```python
from build123d import *

# Parameters (mm, degrees)
F0_W      = 1066.8
F0_H      = 457.2
F1_DEPTH  = 50.8
F2_R      = 50.8
F3_SIZE   = 44.45
F4_W      = 939.8
F4_H      = 330.2
F5_DEPTH  = 25.4
F10_DEPTH = 19.05


with BuildPart() as f1:
    # F0 (on Top) → F1 (new body)
    with BuildSketch(Plane.XY):
        Rectangle(F0_W, F0_H)
    extrude(amount=-F1_DEPTH)

    # F2
    f2_edges = [f1.edges().sort_by_distance(p)[0] for p in [
        (-533.4, -228.6, -25.4),
        (-533.4, 228.6, -25.4),
        (533.4, -228.6, -25.4),
        (533.4, 228.6, -25.4),
    ]]
    fillet(f2_edges, radius=F2_R)

    # F3
    f3_edges = [f1.edges().sort_by_distance(p)[0] for p in [
        (533.4, 0, -50.8),
    ]]
    chamfer(f3_edges, length=F3_SIZE)

    # F4 (on face) → F5 (cut)
    with BuildSketch(Plane(origin=(0, 0, -50.8), x_dir=(1, 0, 0), z_dir=(0, 0, -1))):
        Rectangle(F4_W, F4_H)
    extrude(amount=-F5_DEPTH, mode=Mode.SUBTRACT)

    # F9 (on face) → F10 (join, symmetric)
    with BuildSketch(Plane(origin=(-38.1, 65.991136, 0), x_dir=(0.866025, 0.5, 0), z_dir=(0.5, -0.866025, 0))):
        Polygon((-409.78602, -736.6), (-284.382272, -25.4), (-385.982272, -25.4), (-460.58602, -736.6), align=None)
    extrude(amount=F10_DEPTH, both=True)

    # F11: F1 across plane


with BuildPart() as f1_1:
    add(f1.part)
    add(f1.part.mirror(Plane.YZ))

    # F12: F1 across plane


with BuildPart() as f1_2:
    add(f1_1.part)
    add(f1_1.part.mirror(Plane.XZ))


solid = f1_2.part
```
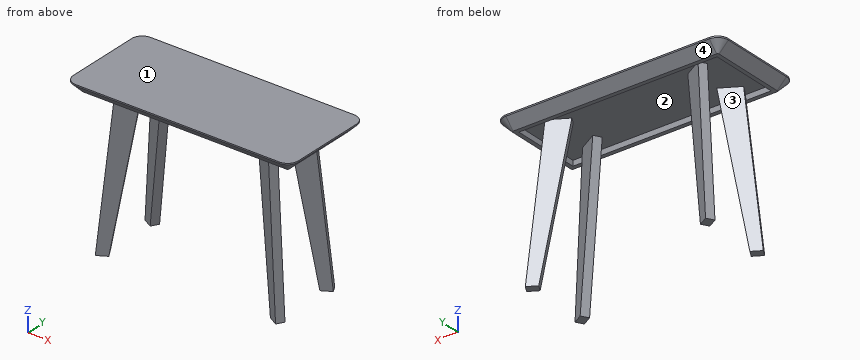
Geometry check sheet. Reference: the model listing, model coordinates, mm. Face numbers are marked on the shaded views. Give positions to 0.01 mm unless a question says otherwise; leave off trailing zeros. Write each loop counter-clockwise with the first axis right and the second up, starting at its lowest first coordinate (ties: lowest second). Pieces come first, ordered by that corner, then holes.
1) Section check D-D, the plane z = -508.5. Record the boundary of the cut face in (x, y).
2) Gauge pin test, flat ends, axial feed: pin 1 (10 mm diameter, centred on y = 115, z = -318, fed in from +X); pin 2 (20.5 mm diameter, centred on x = 157.5, z = -41, fed in from -Y); pin 3 (10 mm diameter, centred on y = -112, z = -191.5, fed in from +X). Record the tip position at first contact, or that the pin passes through.
3) Material ranges on L1, parallel to X at y = -80.5, z = -36; L2, parallel to Z at x = -213.5, y = -13.5; L3, parallel to X at y = 154.5, z = -322, recorded low to high.
4) Section check A-A, the plane x = 193.5. Record the boundary of the cut face in (y, z), and give its area (3 significant figures).
5) Section check B-B, the plane z = -263. Record the boundary of the cut face in (x, y), and give its area (3 significant figures).
6) Section check C-C, the plane y = 33.5. Record the boundary of the cut face in (x, z), and give its area (3 significant figures).
7) Release check for a two-part mould opening along Y. For the marked faces 1, 2, 3 and 4 record: pulls with the +Y half, pulls with the -Y half, needs draft (parallel to the pull), parting line crosses it, or undercut.
Computed:
1. outline: (-425.78, -135.84) - (-406.73, -168.84) - (-348.63, -135.29) - (-367.68, -102.29) - close; (-425.78, 135.84) - (-367.68, 102.29) - (-348.63, 135.29) - (-406.73, 168.84) - close; (348.63, -135.29) - (406.73, -168.84) - (425.78, -135.84) - (367.68, -102.29) - close; (348.63, 135.29) - (367.68, 102.29) - (425.78, 135.84) - (406.73, 168.84) - close
2. pin 1: stops at x = 398.35
2. pin 2: stops at y = -204.2
2. pin 3: stops at x = 393.15
3. L1: x = -503.75 to -469.9, -329.93 to -284.06, 284.06 to 329.93, 469.9 to 503.75
3. L2: z = -25.4 to 0
3. L3: x = -392.42 to -381.9, 381.9 to 392.42
4. outline: (-228.6, -6.35) - (-184.15, -50.8) - (-165.1, -50.8) - (-165.1, -25.4) - (165.1, -25.4) - (165.1, -50.8) - (184.15, -50.8) - (228.6, -6.35) - (228.6, 0) - (-228.6, 0) - close
4. area: 12,900 mm2
5. outline: (-403.48, -122.96) - (-384.43, -155.96) - (-311.14, -113.65) - (-330.19, -80.65) - close; (-403.48, 122.96) - (-330.19, 80.65) - (-311.14, 113.65) - (-384.43, 155.96) - close; (311.14, -113.65) - (384.43, -155.96) - (403.48, -122.96) - (330.19, -80.65) - close; (311.14, 113.65) - (330.19, 80.65) - (403.48, 122.96) - (384.43, 155.96) - close
5. area: 12,900 mm2
6. outline: (-533.4, -6.35) - (-488.95, -50.8) - (-469.9, -50.8) - (-469.9, -25.4) - (469.9, -25.4) - (469.9, -50.8) - (488.95, -50.8) - (533.4, -6.35) - (533.4, 0) - (-533.4, 0) - close
6. area: 28,300 mm2
7. face 1: needs draft
7. face 2: undercut
7. face 3: undercut
7. face 4: pulls with the +Y half
